from build123d import *

# Parameters (mm, degrees)
F0_W        = 57
F0_H        = 20.3
F1_DEPTH    = 44.5
F2_W        = 57
F2_H        = 14.3
F3_DEPTH    = 41.5
F4_R        = 7.62
F5_T1_DEPTH = 265.7262717185
F7_R        = 4
F8_DEPTH    = 25.4
F10_D       = 8
F12_D       = 8
F14_DEPTH   = 25.4
F15_R       = 3.81


# Not quite as in the source:
# - a fillet or chamfer that OpenCascade refuses, or shapes differently, is made with other operations: its cross-section is extruded or revolved along the edge and cut away or added
# - a feature of the source that left no trace in its solid (it failed there, or was rolled back) is left out


with BuildPart() as f1:
    # F0 (on Top) → F1 (new body)
    with BuildSketch(Plane.XY):
        with Locations((0.0714529306, -15.5075108656)):
            Rectangle(F0_W, F0_H)
    extrude(amount=F1_DEPTH)

    # F2 (on face) → F3 (cut)
    with BuildSketch(Plane.XY.offset(44.5)):
        with Locations((0.0714529306, -15.5075108656)):
            Rectangle(F2_W, F2_H)
    extrude(amount=-F3_DEPTH, mode=Mode.SUBTRACT)

    # F4
    f4_edges = [f1.edges().sort_by_distance(p)[0] for p in [
        (-28.428547, -24.157511, 44.5),
        (-28.428547, -6.857511, 44.5),
    ]]
    fillet(f4_edges, radius=F4_R)

    # F5: chamfer of 31.75 x 50.8106212971 on 1 edges, made by hand

    # F5_s2 → F5_t1 (cut)
    with BuildSketch(Plane.XZ.offset(-108.7056249936)):
        Polygon((28.5714529306, 12.75), (-22.2391683665, 44.5), (28.5714529306, 44.5), align=None)
    extrude(amount=F5_T1_DEPTH, mode=Mode.SUBTRACT)

    # F7 (on face) → F8 (cut)
    with BuildSketch(Plane.XZ.offset(25.6575108656)):
        with Locations((-20.8085470694, 36.88)):
            Circle(F7_R)
    extrude(amount=-F8_DEPTH, mode=Mode.SUBTRACT)

    # F10 (through all)
    with Locations(Plane.XY.offset(3)):
        with Locations((18.9828891307, -15.5075108656)):
            Hole(F10_D / 2)

    # F12 (through all)
    with Locations(Plane.XY.offset(3)):
        with Locations((-13.3028933778, -15.5075108656)):
            Hole(F12_D / 2)

    # F13 (on face) → F14 (cut)
    with BuildSketch(Plane.XY.offset(3)):
        with BuildLine():
            Line((-28.4285470694, -19.4970791591), (-13.5915884278, -19.4970791591))
            ThreePointArc((-13.5915884278, -19.4970791591), (-17.3028933778, -15.5075108656), (-13.5915884278, -11.5179425722))
            Line((-13.5915884278, -11.5179425722), (-13.5915884278, -11.4970791591))
            Line((-13.5915884278, -11.4970791591), (-28.4285470694, -11.4970791591))
            Line((-28.4285470694, -11.4970791591), (-28.4285470694, -19.4970791591))
        make_face()
    extrude(amount=-F14_DEPTH, mode=Mode.SUBTRACT)

    # F15
    f15_edges = [f1.edges().sort_by_distance(p)[0] for p in [
        (-22.070718, -24.157511, 44.39474),
        (-22.070718, -6.857511, 44.39474),
    ]]
    fillet(f15_edges, radius=F15_R)


solid = f1.part
Model file for the job. Use its own axes, mm. A direction names the side the tool comes from. Give positions to 0.01 mm unless a question says otherwise; leave off trailing zeros. Loops run counter-clockwise (first coordinate to the right, second up) from the corner with the lowest first, then second, coordinate; pieces in that order, holes last.
1) Saw through at B-B (z = 10). Write the cut outline in (x, y).
2) Pull direction Z, two halves, no side cores. Call faces 4 (the flat face through (-21, -11.497, 2)), 5 (the flat face through (4.34, -6.84, 27.89)), 6 (the cylindrical face through (-24.805, -24.179, 37.056)): +Z half, -Z half, draft (parallel to the pull), parting line (faces both ways), or undercut.
3) Tool access for faces 1 (the flat face through (-21, -19.497, 2)), 2 (the cylindrical face through (-27.4, -6.8, 40.7)), 3 (the flat face through (0, -15, 3)): list every direction of +Z, -Z, +X, -X, +Y, -Y with a clear straight run to the whole face (end or side of a thin tool).
4) Saw through at A-A (y = -7.75). Write the cut outline in (x, z).
5) Saw through at D-D (z = 28.5). Write the cut outline in (x, y), plus the area to 3 significant figures.
6) Wall check: line 1 (Y direction, x = -22.5, z = 9); line 2 (Z direction, x = -5.5, y = -12.5); line 3 (Z direction, x = -22, y = -6.25). Give the ranges that are in metal, low to high.
7) Flat gauge pins, fed straight in: pin 1 Ø5 at (x, y) = (16.5, -9) entering from +Z; pin 2 Ø13 at (x, z) = (-20.81, 36.88) entering from +Y; pin 3 Ø2 at (x, y) = (-12.5, -11) entering from +Z. Where does each tip first touch, or does it go through?
8) Saw through at C-C (x = 4). Write the cut outline in (y, z), plus the area to 3 significant figures.
Answer block:
1. outline: (-28.43, -25.66) - (28.57, -25.66) - (28.57, -22.66) - (-28.43, -22.66) - close; (-28.43, -8.36) - (28.57, -8.36) - (28.57, -5.36) - (-28.43, -5.36) - close
2. face 4: draft
2. face 5: +Z half
2. face 6: undercut
3. face 1: +Z, -Z, -X
3. face 2: +Z, -X, +Y, -Y
3. face 3: +Z, +X, -X
4. outline: (-28.43, 0) - (28.57, 0) - (28.57, 12.75) - (-20.59, 43.47) arc R3.81 ccw to (-24.41, 43.6) arc R7.62 ccw to (-28.43, 36.88) - close; hole circle Ø8 at (-20.81, 36.88)
5. outline: (-28.43, -25.66) - (3.37, -25.66) - (3.37, -22.66) - (-28.43, -22.66) - close; (-28.43, -8.36) - (3.37, -8.36) - (3.37, -5.36) - (-28.43, -5.36) - close
5. area: 191 mm2
6. line 1: y = -25.66 to -22.66, -8.36 to -5.36
6. line 2: z = 0 to 3
6. line 3: z = 0 to 33.06, 40.7 to 44
7. pin 1: stops at z = 21.8
7. pin 2: stops at y = -5.36
7. pin 3: stops at z = 3
8. outline: (-25.66, 0) - (-5.36, 0) - (-5.36, 28.1) - (-8.36, 28.1) - (-8.36, 3) - (-22.66, 3) - (-22.66, 28.1) - (-25.66, 28.1) - close
8. area: 212 mm2
